Read the model definition and answer for the solid it produces. Units are mm, in the model's axes. Face numbers are marked on the shaded views. A direction names the side the tool comes from. Coordinates: 2 decimals unless noted, no trailing zeros. Order: outer loops, then holes, each group sorted by start corner. A loop starts at its lowest first (then second) coordinate and runs counter-clockwise, first axis right, second up. Notation, with made-up numbers: (31, -10.5) - (80, -10.5) arc R23 ccw to (80, 21.5) - close; hole circle Ø3 at (78, -17). An arc over 180 degrees is marked (long way). Write item = value, one per line.
from build123d import *

# Parameters (mm, degrees)
F0_W          = 145
F0_H          = 48
F1_DEPTH      = 15
F0_H_2        = 12
F2_DEPTH      = 15
F4_DEPTH      = 12
F3_R          = 26
F5_DEPTH      = 16
F5_DEPTH_BACK = 4
F3_R_2        = 16
F6_DEPTH      = 21


with BuildPart() as f1:
    # F0 (on Top) → F1 (new body)
    with BuildSketch(Plane.XY):
        with Locations((0, -36)):
            Rectangle(F0_W, F0_H)
        with BuildLine():
            ThreePointArc((-37.5, -43), (-44.5, -36), (-37.5, -29))
            Line((-37.5, -29), (37.5, -29))
            ThreePointArc((37.5, -29), (44.5, -36), (37.5, -43))
            Line((37.5, -43), (-37.5, -43))
        make_face(mode=Mode.SUBTRACT)
    extrude(amount=F1_DEPTH)

    # F0 (on Top) → F2 (join)
    with BuildSketch(Plane.XY):
        with Locations((0, -6)):
            Rectangle(F0_W, F0_H_2)
    extrude(amount=F2_DEPTH)

    # F3 (on Front) → F4 (join)
    with BuildSketch(Plane.XZ):
        with BuildLine():
            Line((-72.5, 15), (-72.5, 0))
            Line((-72.5, 0), (72.5, 0))
            Line((72.5, 0), (72.5, 115))
            ThreePointArc((72.5, 115), (23.030062, 77.431657), (0.121518, 135.171191))
            Line((0.121518, 135.171191), (-72.5, 15))
        make_face()
    extrude(amount=F4_DEPTH)

    # F3 (on Front) → F5 (join, two sides)
    with BuildSketch(Plane.XZ) as f5_sk:
        with BuildLine():
            ThreePointArc((0.121518, 135.171191), (23.030062, 77.431657), (72.5, 115))
            ThreePointArc((72.5, 115), (43.969938, 152.568343), (0.121518, 135.171191))
        make_face()
        with Locations((33.5, 115)):
            Circle(F3_R, mode=Mode.SUBTRACT)
    extrude(amount=F5_DEPTH)
    extrude(f5_sk.sketch, amount=-F5_DEPTH_BACK)

    # F3 (on Front) → F6 (join)
    with BuildSketch(Plane.XZ):
        with Locations((33.5, 115)):
            Circle(F3_R)
        with Locations((33.5, 115)):
            Circle(F3_R_2, mode=Mode.SUBTRACT)
    extrude(amount=F6_DEPTH)


solid = f1.part
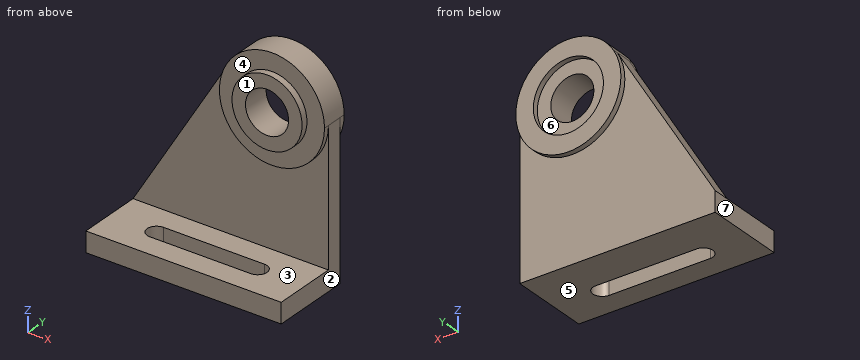
1) For the marked faces 1, 2, 3 and 4, determine the directions among +Z, -Z, +X, -X, +Y, -Y from which every point of the face is accessible in a straight line to the end or side of a thin tool.
Returned:
face_1 = +Z, +X, -X, -Y
face_2 = +Z, -Z, +X, +Y, -Y
face_3 = +X, -X, -Y
face_4 = -Y
2) The part is cut by section A-A (y = -36). Determine the outline of the cut face in (x, z), and give its area (3 significant figures).
Returned:
outline = (-72.5, 0) - (-44.5, 0) - (-44.5, 15) - (-72.5, 15) - close; (44.5, 0) - (72.5, 0) - (72.5, 15) - (44.5, 15) - close
area = 840 mm^2
3) Straight lines are drawn through the part: line 1 along Z through (x, y) = (33, -5); line 2 along Z through (x, y) = (-2.5, -55.5); line 3 along Z through (x, y) = (33.5, 1.8). For each, find the intervals that lie inside material, in ascending order. Write a range as from..to.
Returned:
line_1 = 0..99.01, 130.99..154
line_2 = 0..15
line_3 = 76..89, 141..154
4) Determine the mould class of the marked faces 5, 6 and 7 for opening direction Z: pulls with the +Z half, pulls with the -Z half, needs draft (parallel to the pull), parting line crosses it, or undercut.
Returned:
face_5 = pulls with the -Z half
face_6 = undercut
face_7 = needs draft
5) The part is cut by section D-D (x = 33.5). Determine the outline of the cut face in (y, z), and give its area (3 significant figures).
Returned:
outline = (-60, 0) - (-43, 0) - (-43, 15) - (-60, 15) - close; (-29, 0) - (0, 0) - (0, 76) - (4, 76) - (4, 89) - (0, 89) - (0, 99) - (-21, 99) - (-21, 89) - (-16, 89) - (-16, 76) - (-12, 76) - (-12, 15) - (-29, 15) - close; (-21, 131) - (0, 131) - (0, 141) - (4, 141) - (4, 154) - (-16, 154) - (-16, 141) - (-21, 141) - close
area = 2,360 mm^2
6) The part is cut by section C-C (y = -18). Determine the outline of the cut face in (x, z).
Returned:
outline = (-72.5, 0) - (72.5, 0) - (72.5, 15) - (-72.5, 15) - close; circle Ø52 at (33.5, 115); hole circle Ø32 at (33.5, 115)
7) The part is cut by section B-B (z = 11). Determine the outline of the cut face in (x, y), and give its area (3 significant figures).
Returned:
outline = (-72.5, -60) - (72.5, -60) - (72.5, 0) - (-72.5, 0) - close; hole (-37.5, -43) - (37.5, -43) arc R7 ccw to (37.5, -29) - (-37.5, -29) arc R7 ccw to start
area = 7,500 mm^2
8) Flat-ended cylindrical pins translate along their axes: pin 1 Ø1 at (x, z) = (-8, 124) entering from +Y; pin 2 Ø1 at (x, z) = (-31.5, 32.5) entering from +Y; pin 3 Ø10 at (x, y) = (10, -50.5) entering from +Z. Find the tip coordinate at first contact, or state that the pin passes through.
Returned:
pin_1 = through
pin_2 = 0
pin_3 = 15
